The drawing under review shows one solid part. Ordinate dimensions are in mm from its lowest x, y, z. Coordinates: 2 decimals unless noted, no trailing zeros. Order: outer loops, then holes, each group sorted by start corner. A loop starts at its lowest first (then second) coordinate and runs counter-clockwise, first axis right, second up. Notation, with made-up numbers: (-26, -24) -> (-21, -24) arc R17 ccw to (-21, -18) -> close; hole circle Ø9 at (60.5, -8). An arc over 180 degrees is marked (long way). Use a Markdown table: item, result. Add a question column.
Q1. Wall thickness on probe 1 along X at (y, z) = (1.85, 90); probe 2 along Z at (x, y) = (10, 1.05); probe 3 along X at (y, z) = (2.4, 50): over which ranges is each line inside the solid? List them lowest first.
Q2. Add section D-D (x = 75). State the section outline as (y, z) points, then the cut area to 3 significant figures.
Q3. Add section A-A (x = 140). State the section outline as (y, z) points.
Q4. Add section B-B (z = 70). State the section outline as (x, y) points.
Q5. Add section C-C (y = 1.55). Count the separate pieces of the cut face and the enclosed holes in it, then the cut area to 3 significant figures.
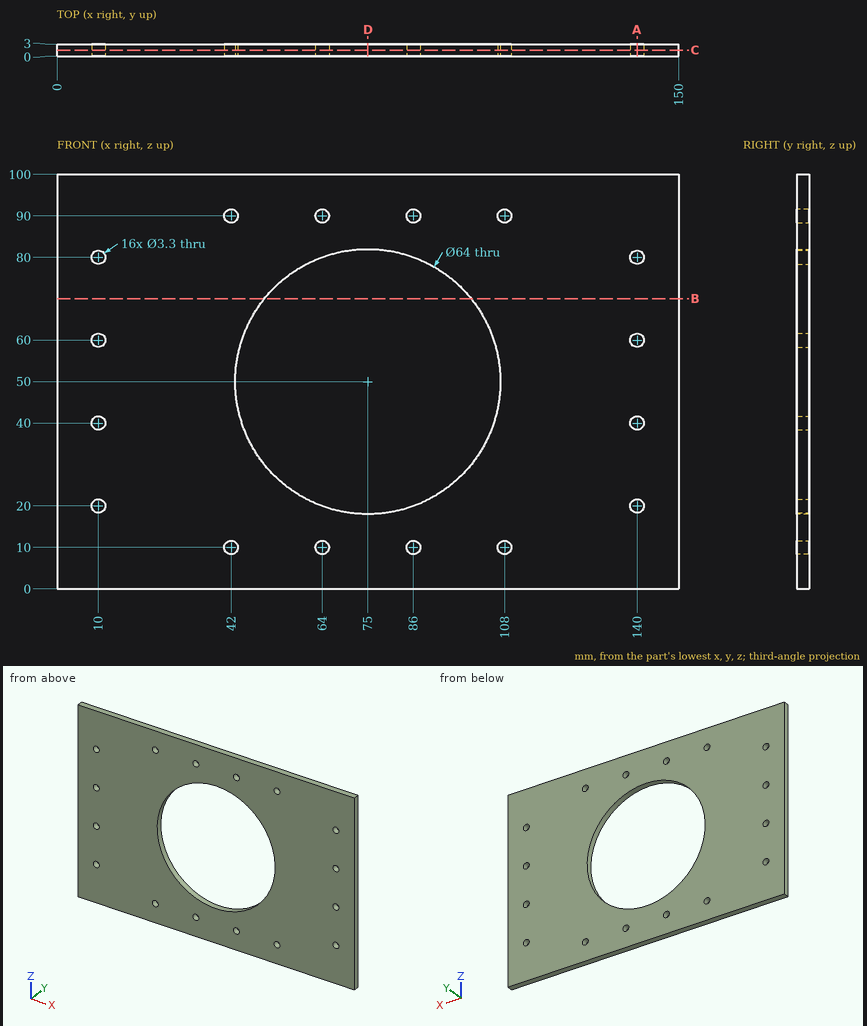
Established:
| question | item | result |
|---|---|---|
| 1 | probe 1 | 0 to 40.35, 43.65 to 62.35, 65.65 to 84.35, 87.65 to 106.35, 109.65 to 150 |
| 1 | probe 2 | 0 to 18.35, 21.65 to 38.35, 41.65 to 58.35, 61.65 to 78.35, 81.65 to 100 |
| 1 | probe 3 | 0 to 43, 107 to 150 |
| 2 | outline | (0, 0) -> (3, 0) -> (3, 18) -> (0, 18) -> close; (0, 82) -> (3, 82) -> (3, 100) -> (0, 100) -> close |
| 2 | area | 108 mm^2 |
| 3 | outline | (0, 0) -> (3, 0) -> (3, 18.35) -> (0, 18.35) -> close; (0, 21.65) -> (3, 21.65) -> (3, 38.35) -> (0, 38.35) -> close; (0, 41.65) -> (3, 41.65) -> (3, 58.35) -> (0, 58.35) -> close; (0, 61.65) -> (3, 61.65) -> (3, 78.35) -> (0, 78.35) -> close; (0, 81.65) -> (3, 81.65) -> (3, 100) -> (0, 100) -> close |
| 4 | outline | (0, 0) -> (50.02, 0) -> (50.02, 3) -> (0, 3) -> close; (99.98, 0) -> (150, 0) -> (150, 3) -> (99.98, 3) -> close |
| 5 | separate pieces | 1 |
| 5 | enclosed holes | 17 |
| 5 | area | 11,600 mm^2 |
